CAD build for the part. Positions are in the model's coordinates, mm. Give positions to 0.01 mm unless a question says otherwise; leave off trailing zeros. Write each loop counter-clockwise with the first axis right and the second up, starting at its lowest first coordinate (ties: lowest second). Pieces come first, ordered by that corner, then holes. Notation, with made-up numbers: (15, 65.5) - (60, 65.5) arc R13 cw to (60, 85.5) - close; hole circle Ø1 at (9.5, 70). An arc over 180 degrees is marked (long way). Answer as a JSON object with one key per item and string values.
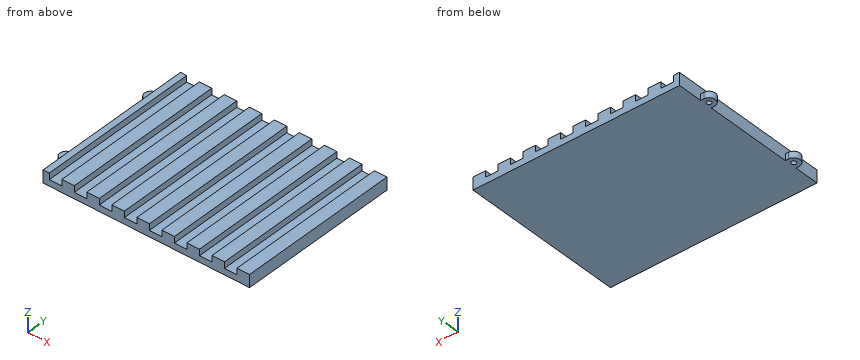
from build123d import *

# Parameters (mm, degrees)
F1_DEPTH = 165.1
F2_R     = 2.3876
F3_DEPTH = 6.35


with BuildPart() as f1:
    # F0 (on Front) → F1 (new body)
    with BuildSketch(Plane.XZ):
        Polygon((-104.775, 12.7), (-104.775, 0), (104.775, 0), (104.775, 12.7), (92.075, 12.7), (92.075, 6.35), (79.375, 6.35), (79.375, 12.7), (66.675, 12.7), (66.675, 6.35), (53.975, 6.35), (53.975, 12.7), (41.275, 12.7), (41.275, 6.35), (28.575, 6.35), (28.575, 12.7), (15.875, 12.7), (15.875, 6.35), (3.175, 6.35), (3.175, 12.7), (-9.525, 12.7), (-9.525, 6.35), (-22.225, 6.35), (-22.225, 12.7), (-34.925, 12.7), (-34.925, 6.35), (-47.625, 6.35), (-47.625, 12.7), (-60.325, 12.7), (-60.325, 6.35), (-73.025, 6.35), (-73.025, 12.7), (-85.725, 12.7), (-85.725, 6.35), (-98.425, 6.35), (-98.425, 12.7), align=None)
    extrude(amount=F1_DEPTH)

    # F2 (on face) → F3 (join)
    with BuildSketch(Plane(origin=(0, 0, 0), x_dir=(1, 0, 0), z_dir=(0, 0, -1))):
        with BuildLine():
            Line((-107.95, 25.4), (-104.775, 25.4))
            Line((-104.775, 25.4), (-104.775, 38.1))
            Line((-104.775, 38.1), (-107.95, 38.1))
            ThreePointArc((-107.95, 38.1), (-114.3, 31.75), (-107.95, 25.4))
        make_face()
        with Locations((-107.95, 31.75)):
            Circle(F2_R, mode=Mode.SUBTRACT)
        with BuildLine():
            ThreePointArc((-107.95, 139.7), (-114.3, 133.35), (-107.95, 127))
            Line((-107.95, 127), (-104.775, 127))
            Line((-104.775, 127), (-104.775, 139.7))
            Line((-104.775, 139.7), (-107.95, 139.7))
        make_face()
        with Locations((-107.95, 133.35)):
            Circle(F2_R, mode=Mode.SUBTRACT)
    extrude(amount=-F3_DEPTH)


solid = f1.part
(1) Saw through at A-A, the plane z = 8.75. State how many separate pieces and enclosed holes the cut face has, and give its area (3 significant figures).
Answer key:
{"separate pieces": "9", "enclosed holes": "0", "area": "17,800 mm²"}
(2) Saw through at B-B, the plane x = 88.5. Give the cut face in (y, z).
Answer key:
{"outline": "(-165.1, 0) - (0, 0) - (0, 6.35) - (-165.1, 6.35) - close"}
(3) Flat gauge pins, fed straight in: P1, Ø1.6, axis at x = -107, z = 2.5, coming from the -Y side; P2, Ø1.9, axis at y = -102.5, z = 8.5, coming from the -X side (3 decimals); P3, Ø4, axis at x = -95, y = -72, coming from the +Z side; P4, Ø2, axis at x = 77.5, z = 6, coming from the +Y side. Where does each tip first touch, or does it go through?
Answer key:
{"P1": "stops at y = -139.7", "P2": "stops at x = -104.775", "P3": "stops at z = 6.35", "P4": "stops at y = 0"}
(4) Probe L1, parallel to Y at x = -107.95, z = 5; L2, parallel to X at y = -133.35, z = 3.25 (3 decimals); L3, parallel to X at y = -108, z = 4.5 (3 decimals). List the from-to ranges inside material, lowest first. Write a range as [from, to].
Answer key:
{"L1": "y = [-139.7, -135.74], [-130.96, -127], [-38.1, -34.14], [-29.36, -25.4]", "L2": "x = [-114.3, -110.338], [-105.562, 104.775]", "L3": "x = [-104.775, 104.775]"}
